Geometry: final body of the model. Coordinates: model frame, mm. A direction names the side the tool comes from. Coordinates: 2 decimals unless noted, no trailing zeros. Write each loop counter-clockwise with the first axis right and the second up, starting at its lowest first coordinate (ties: lowest second). Pieces come first, ordered by that corner, then holes. Notation, with made-up numbers: (26.5, -27.5) -> (44.5, -27.5) arc R8 ccw to (44.5, -21.5) -> close; hole circle Ø4 at (84.25, 85). An arc over 180 degrees is marked (long way). Answer as a JSON object with one key per item and string values. Group by question number.
```python
from build123d import *

# Parameters (mm, degrees)
PRISM_DEPTH       = 2
CYLINDER013_R     = 2.7
CYLINDER013_DEPTH = 3


with BuildPart() as prism:
    # Prism → Prism (new body)
    with BuildSketch(Plane.XY.offset(-23)):
        Polygon((1.4, 0), (0.7, 1.212436), (-0.7, 1.212436), (-1.4, 0), (-0.7, -1.212436), (0.7, -1.212436), align=None)
    extrude(amount=PRISM_DEPTH)


with BuildPart() as cut008:
    # Cylinder013 → Cylinder013 (new body)
    with BuildSketch(Plane.XY.offset(-23)):
        Circle(CYLINDER013_R)
    extrude(amount=CYLINDER013_DEPTH)

    # Cut008: cut Prism
    add(prism.part, mode=Mode.SUBTRACT)


solid = cut008.part
```
Item 1: Ray query, L1, parallel to X at y = -0.8, z = -21.7; L2, parallel to Z at x = 0.9, y = -0.6; L3, parallel to X at y = 0.75, z = -21.35. Return the intervals inside material, ascending. Write a range as [from, to].
Item 2: Section A-A on z = -21.85. Output: boundary loops of the cut face in (x, y), then the cut area to 3 significant figures.
Item 3: Mould query, pull axis X, two halves, no side actions, for faces 3 (the cylindrical face through (-0.585, -2.636, -21.521)), 4 (the flat face through (0, 0, -21)), 5 (the flat face through (1, -1, -23)). Classes: +X half, -X half, draft (parallel to the pull), parting line (faces both ways), or undercut.
Item 4: Set-up query: faces 1 (the flat face through (0, 0, -20)), 2 (the flat face through (1.05, -0.61, -22.01)). Return all of +Z, -Z, +X, -X, +Y, -Y with unobstructed straight access to the full face (end or side cutting, diameter ignored); none if empty.
Item 5: Section B-B on x = 0. Output: boundary loops of the cut face in (y, z), then the cut area to 3 significant figures.
Item 6: Section C-C on y = 0.2. Output: boundary loops of the cut face in (x, z).
Item 7: Section D-D on z = -20.8. Output: boundary loops of the cut face in (x, y).
Answer sheet:
{
 "1": {"L1": "x = [-2.58, -0.94], [0.94, 2.58]", "L2": "z = [-21, -20]", "L3": "x = [-2.59, -0.97], [0.97, 2.59]"},
 "2": {"outline": "circle Ø5.4 at (0, 0); hole (-1.4, 0) -> (-0.7, -1.21) -> (0.7, -1.21) -> (1.4, 0) -> (0.7, 1.21) -> (-0.7, 1.21) -> close", "area": "17.8 mm^2"},
 "3": {"face 3": "parting line", "face 4": "undercut", "face 5": "draft"},
 "4": {"face 1": "+Z, +X, -X, +Y, -Y", "face 2": "-Z"},
 "5": {"outline": "(-2.7, -23) -> (-1.21, -23) -> (-1.21, -21) -> (1.21, -21) -> (1.21, -23) -> (2.7, -23) -> (2.7, -20) -> (-2.7, -20) -> close", "area": "11.4 mm^2"},
 "6": {"outline": "(-2.69, -23) -> (-1.28, -23) -> (-1.28, -21) -> (1.28, -21) -> (1.28, -23) -> (2.69, -23) -> (2.69, -20) -> (-2.69, -20) -> close"},
 "7": {"outline": "circle Ø5.4 at (0, 0)"}
}
